Autodesk Inventor part; units mm, degrees
ref_plane "YZ Plane" through (0, 0, 0) normal (1, 0, 0) x (0, 1, 0)
ref_plane "XZ Plane" through (0, 0, 0) normal (0, 1, 0) x (-1, 0, 0)
ref_plane "XY Plane" through (0, 0, 0) normal (0, 0, 1) x (1, 0, 0)
sketch "Sketch1" plane through (0, 0, 0) normal (0, 0, 1) x (1, 0, 0)
  circle A0 centre (-45.0744, 20) radius 1.4
  circle A1 centre (-45, 5.0002) radius 1.4
  line L0 (-55, 0) -> (-55, 35)
  line L1 (-55, 25) -> (-46.5743, 25)
  line L2 (-46.5743, 25) -> (-40.0744, 18.5001)
  line L3 (-40.0744, 18.5001) -> (-40.0744, 6.5001)
  line L4 (-40.0744, 6.5001) -> (-46.5743, 0.0002)
  line L5 (-46.5743, 0.0002) -> (-55, 0.0002)
  point P0 (0, 0)
  point P1 (-50.7872, 0.0002)
  dimension "d0" = 5
  dimension "d1" = 5
  dimension "d2" = 45
  dimension "d3" = 5
  dimension "d4" = 12
extrude "Extrusion1" add sketch "Sketch1" along normal blind 4
sketch "Sketch2" plane through (-55, 0.0002, 0) normal (-1, 0, 0) x (0, 0, 1)
  line L0 (0, 24.9998) -> (0, 0)
  line L1 (0, 0) -> (4, 0)
  line L2 (4, 24.9998) -> (4, 0)
  line L3 (0, 24.9998) -> (4, 24.9998)
  line L4 (4, 18.4999) -> (4, 24.9998)
  line L5 (4, 24.9998) -> (28, 24.9998)
  line L6 (28, 24.9998) -> (28, 0)
  line L7 (4, 24.9998) -> (4, 0)
  line L8 (28, 0) -> (4, 0)
  point P0 (0, -0.0002)
  dimension "d7" = 24
extrude "Extrusion2" add sketch "Sketch2" against normal blind 2 contours L5 L6 L8 L2
sketch "Sketch4" plane through (-55, 0.0002, 0) normal (0, -1, 0) x (1, 0, 0)
  line L0 (2, 28) -> (2, 4)
  line L1 (2, 4) -> (8.4257, 4)
  line L2 (8.4257, 0) -> (8.4257, 4)
  line L3 (2, 4) -> (2, 28)
  line L4 (8.4257, 4) -> (2, 28)
  point P0 (55, 0)
extrude "Extrusion4" add sketch "Sketch4" against normal blind 2
sketch "Sketch5" plane through (-55, 0.0002, 0) normal (-1, 0, 0) x (0, 0, 1)
  line L0 (0, 24.9998) -> (0, 0)
  line L1 (0, 0) -> (28, 0)
  line L2 (28, 0) -> (28, 24.9998)
  line L3 (0, 24.9998) -> (28, 24.9998)
  point P0 (0, -0.0002)
  point P1 (20.5, 19)
  point P2 (20.5, 9)
  point P3 (13.5, 9)
  point P4 (13.5, 19)
  dimension "d14" = 9
  dimension "d15" = 7
  dimension "d16" = 10
  dimension "d17" = 7.5
hole "Hole1" at (-55, 19.0002, 20.5) at (-55, 9.0002, 20.5) at (-55, 9.0002, 13.5) at (-55, 19.0002, 13.5) direction (1, 0, 0) diameter 2.8 end through all
equation "\"d1\" = d0"
properties part number "Drag Chain Base" material "ABS Plastic"
Model file for the job. Use its own axes, mm. A direction names the side the tool comes from. Coordinates: 2 decimals unless noted, no trailing zeros. Order: outer loops, then holes, each group sorted by start corner. A loop starts at its lowest first (then second) coordinate and runs counter-clockwise, first axis right, second up. Notation, with made-up numbers: (-8, 85.25) - (35, 85.25) arc R13 cw to (35, 95.25) - close; hole circle Ø9 at (22.25, 50). An arc over 180 degrees is marked (long way). Return JSON: item names as keys, results as strings. Group by question number.
1) Saw through at B-B, the plane y = 20. Write the cut outline in (x, z), plus the area to 3 significant figures.
2) Saw through at A-A, the plane z = 13.75. Write the cut outline in (x, y), plus the area to 3 significant figures.
3) Flat gauge pins, fed straight in: P1, Ø1.5, axis at y = 17.5, z = 9.5, coming from the +X side; P2, Ø4, axis at x = -46.5, y = 16.5, coming from the +Z side; P3, Ø1.9, axis at x = -49.5, z = 21, coming from the +Y side; P4, Ø1, axis at x = -45.5, z = 4, coming from the -Y side. Where does each tip first touch, or does it go through?
4) Saw through at C-C, the plane x = -45. Write the cut outline in (y, z), plus the area to 3 significant figures.
5) Saw through at D-D, the plane z = 2.25. Write the cut outline in (x, y).
6) Probe line 1 (Y direction, x = -54.2, z = 13.5); line 2 (Y direction, x = -45, z = 2.65); line 3 (X direction, y = 7, z = 6.25). List the from-to ranges inside material, lowest first. Write a range as from..to.
7) Mould opens along Y. For faces 3 (the flat face through (-51, 2, 11)), 4 (the flat face through (-54, 13, 28)), 5 (the cylindrical face through (-43.71, 5.54, 1.97)) say: released by +Y, released by -Y, zero draft, split by the parting line, or undercut.
8) Tool access for faces 1 (the flat face through (-47, 13, 4)), 2 (the cylindrical face through (-53.99, 8.94, 12.1)): list every direction of +Z, -Z, +X, -X, +Y, -Y with a clear straight run to the whole face (end or side of a thin tool).
Values found:
{
 "1": {"outline": "(-55, 0) - (-46.47, 0) - (-46.47, 4) - (-53, 4) - (-53, 12.52) - (-55, 12.52) - close; (-55, 14.48) - (-53, 14.48) - (-53, 19.52) - (-55, 19.52) - close; (-55, 21.48) - (-53, 21.48) - (-53, 28) - (-55, 28) - close; (-43.67, 0) - (-41.57, 0) - (-41.57, 4) - (-43.67, 4) - close", "area": "82.7 mm²"},
 "2": {"outline": "(-55, 0) - (-49.18, 0) - (-49.18, 2) - (-53, 2) - (-53, 7.62) - (-55, 7.62) - close; (-55, 10.38) - (-53, 10.38) - (-53, 17.62) - (-55, 17.62) - close; (-55, 20.38) - (-53, 20.38) - (-53, 25) - (-55, 25) - close", "area": "46.6 mm²"},
 "3": {"P1": "stops at x = -53", "P2": "stops at z = 4", "P3": "passes through", "P4": "stops at y = 0.57"},
 "4": {"outline": "(1.57, 0) - (3.6, 0) - (3.6, 4) - (1.57, 4) - close; (6.4, 0) - (18.6, 0) - (18.6, 4) - (6.4, 4) - close; (21.4, 0) - (23.43, 0) - (23.43, 4) - (21.4, 4) - close", "area": "65.0 mm²"},
 "5": {"outline": "(-55, 0) - (-46.57, 0) - (-40.07, 6.5) - (-40.07, 18.5) - (-46.57, 25) - (-55, 25) - close; hole circle Ø2.8 at (-45.07, 20); hole circle Ø2.8 at (-45, 5)"},
 "6": {"line 1": "y = 0..7.6, 10.4..17.6, 20.4..25", "line 2": "y = 1.57..3.6, 6.4..18.6, 21.4..23.43", "line 3": "x = -55..-53"},
 "7": {"face 3": "released by +Y", "face 4": "zero draft", "face 5": "undercut"},
 "8": {"face 1": "+Z, +X, +Y", "face 2": "+X, -X"}
}
